Autodesk Inventor part; units mm, degrees
ref_plane "Work Plane1" through (-68.5, 0, 0) normal (1, 0, 0) x (0, 0, -1)
ref_plane "YZ Plane" through (0, 0, 0) normal (1, 0, 0) x (0, 1, 0)
ref_plane "XZ Plane" through (0, 0, 0) normal (0, 1, 0) x (-1, 0, 0)
sketch "Sketch1" plane through (0, 0, 0) normal (0, 0, 1) x (1, 0, 0)
  line L0 (0, 0) -> (-137, 0)
  line L1 (-137, 0) -> (-137, 160)
  line L2 (-137, 160) -> (0, 160)
  line L3 (0, 160) -> (0, 0)
  dimension "d0" = 137
  dimension "d1" = 160
extrude "Extrusion1" add sketch "Sketch1" along normal blind 82
sketch "Sketch2" plane through (0, 0, 82) normal (0, 0, 1) x (1, 0, 0)
  line L0 (-7, 11) -> (-130, 11)
  line L1 (-130, 11) -> (-130, 153)
  line L2 (-130, 153) -> (-7, 153)
  line L3 (-7, 153) -> (-7, 11)
  line L4 (-137, 160) -> (-137, 0)
  line L5 (0, 0) -> (0, 160)
  line L6 (0, 160) -> (-137, 160)
  line L7 (-137, 0) -> (0, 0)
  dimension "d4" = 7
  dimension "d5" = 7
  dimension "d6" = 7
  dimension "d7" = 11
extrude "Extrusion2" cut sketch "Sketch2" against normal blind 78 contours L0 L1 L2 L3
sketch "Sketch3" plane through (0, 0, 82) normal (0, 0, 1) x (1, 0, 0)
  line L0 (-7, 11) -> (-130, 11)
  line L1 (-130, 11) -> (-123.6491, 0)
  line L2 (0, 0) -> (-137, 0)
  line L3 (-130, 11) -> (-117.2983, 11) construction
  line L4 (-7, 11) -> (-13.3509, 0)
  line L5 (-7, 11) -> (5.7017, 11) construction
  line L6 (-13.3509, 0) -> (-123.6491, 0)
  line L7 (-130, 11) -> (-7, 11)
  dimension "d10" = 60
  dimension "d11" = 120
extrude "Extrusion3" cut sketch "Sketch3" against normal blind 40
sketch "Sketch4" plane through (-137, 0, 0) normal (-1, 0, 0) x (0, 0, 1)
  line L0 (73, 160) -> (9, 160)
  line L1 (9, 160) -> (9, 25)
  line L2 (9, 25) -> (73, 25)
  line L3 (73, 25) -> (73, 160)
  line L4 (82, 160) -> (82, 0)
  line L5 (0, 0) -> (0, 160)
  line L6 (0, 160) -> (82, 160)
  line L7 (0, 0) -> (82, 0)
  dimension "d14" = 9
  dimension "d15" = 9
  dimension "d16" = 0
  dimension "d17" = 25
extrude "Extrusion4" cut sketch "Sketch4" against normal blind 5 contours L3 L2 L1 L0
ref_plane "Work Plane1" through (-68.5, 0, 0) normal (1, 0, 0) x (0, 0, -1)
mirror "Mirror1" about plane through (-68.5, 0, 0) normal (1, 0, 0) of "Extrusion4"
sketch "Sketch5" plane through (-137, 160, 0) normal (0, 1, 0) x (1, 0, 0)
  line L0 (137, -73) -> (132, -73)
  line L1 (5, -73) -> (5, -9)
  line L2 (132, -73) -> (5, -73)
  line L3 (5, -73) -> (5, -9)
  line L4 (5, -9) -> (132, -9)
  line L5 (132, -9) -> (132, -73)
  point P0 (137, 0)
extrude "Extrusion5" cut sketch "Sketch5" against normal blind 5
fillet "Fillet1" radius 15 1 edges at (-68.5, 11, 4)
fillet "Fillet2" radius 15 1 edges at (-68.5, 0, 0)
sketch "Sketch6" plane through (-137, 0, 82) normal (-1, 0, 0) x (0, 0, 1)
  circle A0 centre (0, -50) radius 65
  line L0 (-67, 0) -> (0, 0)
  line L1 (0, 160) -> (0, 0)
  point P0 (-82, 0)
  dimension "d24" = 130
  dimension "d25" = 50
  dimension "d26" = 0
extrude "Extrusion6" cut sketch "Sketch6" against normal through all
fillet "Fillet3" radius 5 2 edges at (-133.5, 15, 82) (-3.5, 15, 82)
properties part number "box"
Here's how the part is built. I have some questions about the finished solid (model axes, mm). A direction names the side the tool comes from. Coordinates: 2 decimals unless noted, no trailing zeros. Write each loop counter-clockwise with the first axis right and the second up, starting at its lowest first coordinate (ties: lowest second). Pieces come first, ordered by that corner, then holes. Notation, with made-up numbers: (-38.5, 13.5) - (17.5, 13.5) arc R21 cw to (17.5, 32.5) - close; hole circle Ø7 at (74.25, -3.75). An arc over 180 degrees is marked (long way). One line per item, written item: value.
1) Suppose I cut it at C-C on x = -39. Write out the boundary of the cut face in (y, z), and give its area (3 significant figures).
Model answer:
outline: (0, 15) arc R15 ccw to (15, 0) - (160, 0) - (160, 9) - (155, 9) - (155, 73) - (160, 73) - (160, 82) - (153, 82) - (153, 4) - (26, 4) arc R15 cw to (11, 19) - (11, 42) - (1.23, 42) arc R65 cw to (0, 40.47) - close
area: 1,280 mm²
2) I need wall thicknesses on line 1 along X through (y, z) = (75.5, 75.5); line 2 along X through (y, z) = (87, 54); line 3 along Y through (x, z) = (-26.5, 29.5). Which ranges of each line are inside material? Lowest first, please.
Model answer:
line 1: x = -137 to -130, -7 to 0
line 2: x = -132 to -130, -7 to -5
line 3: y = 0 to 11, 153 to 155
3) Suppose I cut it at D-D on z = 75. Write out the boundary of the cut face in (x, y), and give its area (3 significant figures).
Model answer:
outline: (-137, 14.62) - (-130, 14.62) - (-130, 153) - (-7, 153) - (-7, 14.62) - (0, 14.62) - (0, 160) - (-137, 160) - close
area: 2,900 mm²
4) I'm going to push flat-ended pins straight in: P1, Ø6, axis at y = 33.5, z = 56.5, coming from the +X side; P2, Ø5, axis at x = -66.5, z = 57, coming from the +Y side; P3, Ø8, axis at y = 32.5, z = 53, coming from the -X side. Where does each tip first touch, or does it pass through?
Model answer:
P1: stops at x = -5
P2: stops at y = 155
P3: stops at x = -132
5) Suppose I cut it at A-A on z = 31. Write out the boundary of the cut face in (x, y), and give its area (3 significant figures).
Model answer:
outline: (-137, 0) - (0, 0) - (0, 25) - (-5, 25) - (-5, 155) - (-132, 155) - (-132, 25) - (-137, 25) - close; hole (-130, 11) - (-7, 11) - (-7, 153) - (-130, 153) - close
area: 2,470 mm²
6) On a 3-axis mill with a long thin cutter (end or side, diameter ignored), from which of +Z, -Z, +X, -X, +Y, -Y can I reach the whole of each face in a straight line? I mean faces 5 (the flat face through (-69, 90, 4)), 6 (the flat face through (-2, 25, 41)), 7 (the flat face through (-135, 25, 41)), 8 (the flat face through (-69, 158, 82)). Say none if no direction works.
Model answer:
face 5: +Z
face 6: +X, +Y
face 7: -X, +Y
face 8: +Z, +X, -X, +Y, -Y
7) Suppose I cut it at B-B on y = 64. Write out the boundary of the cut face in (x, z), and give its area (3 significant figures).
Model answer:
outline: (-137, 0) - (0, 0) - (0, 9) - (-5, 9) - (-5, 73) - (0, 73) - (0, 82) - (-7, 82) - (-7, 4) - (-130, 4) - (-130, 82) - (-137, 82) - (-137, 73) - (-132, 73) - (-132, 9) - (-137, 9) - close
area: 1,000 mm²
8) We'd pull the mould along X, two halves only. Please class faces 1 (the flat face through (-130, 81, 44)), 2 (the flat face through (-132, 91, 41)), 3 (the flat face through (-69, 158, 9)), 4 (the cylindrical face through (-69.36, 15.51, 8.28)): pulls with the +X half, pulls with the -X half, needs draft (parallel to the pull), parting line crosses it, or undercut.
Model answer:
face 1: undercut
face 2: pulls with the -X half
face 3: needs draft
face 4: undercut
